from build123d import *

# Parameters (mm, degrees)
SKETCH1_W           = 66.85
SKETCH1_H           = 96.52
BOSS_EXTRUDE2_DEPTH = 3
SKETCH2_W           = 31.925
SKETCH2_H           = 3
CUT_EXTRUDE1_DEPTH  = 3
SKETCH3_W           = 48.26
SKETCH3_H           = 3
CUT_EXTRUDE2_DEPTH  = 3
SKETCH4_W           = 10.643333334
SKETCH4_H           = 3
BOSS_EXTRUDE3_DEPTH = 3
SKETCH5_W           = 16.086666666
SKETCH5_H           = 3
BOSS_EXTRUDE4_DEPTH = 3
SKETCH6_R           = 1.45
CUT_EXTRUDE10_DEPTH = 3
SKETCH7_R           = 1.45
CUT_EXTRUDE11_DEPTH = 3
SKETCH9_W           = 96.52
SKETCH9_H           = 3
BOSS_EXTRUDE5_DEPTH = 17.25
SKETCH10_W          = 12.7
SKETCH10_H          = 6.86
CUT_EXTRUDE12_DEPTH = 3
SKETCH12_W          = 15
SKETCH12_H          = 3
CUT_EXTRUDE14_DEPTH = 3


with BuildPart() as part:
    # Sketch1 → Boss-Extrude2 (new body)
    with BuildSketch(Plane(origin=(0, 0, 0), x_dir=(1, 0, 0), z_dir=(0, 1, 0))):
        Rectangle(SKETCH1_W, SKETCH1_H)
    extrude(amount=BOSS_EXTRUDE2_DEPTH)

    # Sketch2 → Cut-Extrude1 (cut)
    with BuildSketch(Plane.XY.offset(48.26)):
        with Locations((0, 1.5)):
            Rectangle(SKETCH2_W, SKETCH2_H)
    cut_extrude1 = extrude(amount=-CUT_EXTRUDE1_DEPTH, mode=Mode.SUBTRACT)

    # Mirror1: Cut-Extrude1 across plane
    add(cut_extrude1.mirror(Plane.XY), mode=Mode.SUBTRACT)

    # Sketch3 → Cut-Extrude2 (cut)
    with BuildSketch(Plane.ZY.offset(33.425)):
        with Locations((0, 1.5)):
            Rectangle(SKETCH3_W, SKETCH3_H)
    extrude(amount=-CUT_EXTRUDE2_DEPTH, mode=Mode.SUBTRACT)

    # Sketch4 → Boss-Extrude3 (add)
    with BuildSketch(Plane.XY.offset(45.26)):
        with Locations((0, 1.5)):
            Rectangle(SKETCH4_W, SKETCH4_H)
    boss_extrude3 = extrude(amount=BOSS_EXTRUDE3_DEPTH)

    # Mirror2: Boss-Extrude3 across plane
    add(boss_extrude3.mirror(Plane.XY))

    # Sketch5 → Boss-Extrude4 (add)
    with BuildSketch(Plane.ZY.offset(30.425)):
        with Locations((0, 1.5)):
            Rectangle(SKETCH5_W, SKETCH5_H)
    extrude(amount=BOSS_EXTRUDE4_DEPTH)

    # Sketch6 → Cut-Extrude10 (cut)
    with BuildSketch(Plane(origin=(0, 3, 0), x_dir=(1, 0, 0), z_dir=(0, 1, 0))):
        with Locations((-32.075, 0)):
            Circle(SKETCH6_R)
    extrude(amount=-CUT_EXTRUDE10_DEPTH, mode=Mode.SUBTRACT)

    # Sketch7 → Cut-Extrude11 (cut)
    with BuildSketch(Plane(origin=(0, 3, 0), x_dir=(1, 0, 0), z_dir=(0, 1, 0))):
        with Locations((-0.211991592, -46.91)):
            Circle(SKETCH7_R)
    cut_extrude11 = extrude(amount=-CUT_EXTRUDE11_DEPTH, mode=Mode.SUBTRACT)

    # Mirror3: Cut-Extrude11 across plane
    add(cut_extrude11.mirror(Plane.XY), mode=Mode.SUBTRACT)

    # Sketch9 → Boss-Extrude5 (add)
    with BuildSketch(Plane(origin=(33.425, 0, 0), x_dir=(0, 0, -1), z_dir=(1, 0, 0))):
        with Locations((0, 1.5)):
            Rectangle(SKETCH9_W, SKETCH9_H)
    extrude(amount=BOSS_EXTRUDE5_DEPTH)

    # Sketch10 → Cut-Extrude12 (cut)
    with BuildSketch(Plane.XZ):
        with Locations((34.325, 0)):
            Rectangle(SKETCH10_W, SKETCH10_H)
    extrude(amount=-CUT_EXTRUDE12_DEPTH, mode=Mode.SUBTRACT)

    # Sketch12 → Cut-Extrude14 (cut)
    with BuildSketch(Plane.XZ):
        with Locations((38.175, -16.76)):
            Rectangle(SKETCH12_W, SKETCH12_H)
    extrude(amount=-CUT_EXTRUDE14_DEPTH, mode=Mode.SUBTRACT)


solid = part.part
Design review of the part built by this model. Coordinates are the model's own, in mm. A direction names the side the tool comes from. Round coordinates to 2 decimals unless told otherwise and drop trailing zeros. Loops run counter-clockwise (first coordinate to the right, second up) from the corner with the lowest first, then second, coordinate; pieces in that order, holes last. Notation, with made-up numbers: (87, -29.5) -> (135, -29.5) arc R33 ccw to (135, 3.5) -> close; hole circle Ø1 at (58.25, 34.25). An arc over 180 degrees is marked (long way). Use one line per item in the form item = value. Start each with the question number.
Q1. Machinability: for faces 1 (the face through (-32, 1, 8.043)), 2 (the face through (-33.425, 2, -4)), 3 (the face through (15.962, 1, 47)), 4 (the face through (-11, 2, -45.26)), 5 (the face through (30.675, 1, -17)), which of the approach directions +Z, -Z, +X, -X, +Y, -Y give a long, thin tool a straight path to every point of the face, cutting with its end or side? Answer none if there is none.
Q2. For pin 1 Ø1.5 at (y, z) = (2, -13) entering from -X (3 decimals); pin 2 Ø2 at (x, z) = (36.5, 1) entering from +Y; pin 3 Ø1.5 at (x, y) = (10.5, 1) entering from -Z, all flat-tipped, find the tip position at first contact; note any pin that passes through.
Q3. We need section B-B on y = 1.65. State how many separate pieces and enclosed holes the cut face has, then the cut area to 3 significant figures.
Q4. Wall thickness on line 1 along X through (y, z) = (1.8, -46.91) (1 decimal); line 2 along X through (y, z) = (1.6, 0) (3 decimals); line 3 along Z through (x, y) = (33, 1): over which ranges is each line inside the solid? List them lowest first. Write a range as [from, to].
Q5. Draft analysis for pull direction X (two halves, no side actions). For faces 6 (the face through (-25, 1, 48.26)), 7 (the face through (-15.962, 1, -47)), 8 (the face through (-33.425, 1, -36)), state which applies: +X half, -X half, draft (parallel to the pull), parting line (faces both ways), or undercut.
Q6. We need section A-A on z = -46.91. Give the boundary of the cut face in (x, y) (1 decimal), then the cut area to 3 significant figures.
Calculated:
q1.face_1 = -X, +Y, -Y
q1.face_2 = +Z, -Z, -X, +Y, -Y
q1.face_3 = +Z, +Y, -Y
q1.face_4 = -Z, +Y, -Y
q1.face_5 = +Y, -Y
q2.pin_1 = -30.425
q2.pin_2 = through
q2.pin_3 = -45.26
q3.separate_pieces = 1
q3.enclosed_holes = 2
q3.area = 7,740 mm²
q4.line_1 = [-33.4, -16], [-5.3, -1.7], [1.2, 5.3], [16, 50.7]
q4.line_2 = [-30.625, 27.975], [40.675, 50.675]
q4.line_3 = [-48.26, -18.26], [-15.26, -3.43], [3.43, 48.26]
q5.face_6 = draft
q5.face_7 = undercut
q5.face_8 = -X half
q6.outline = (-33.4, 0) -> (-16, 0) -> (-16, 3) -> (-33.4, 3) -> close; (-5.3, 0) -> (-1.7, 0) -> (-1.7, 3) -> (-5.3, 3) -> close; (1.2, 0) -> (5.3, 0) -> (5.3, 3) -> (1.2, 3) -> close; (16, 0) -> (50.7, 0) -> (50.7, 3) -> (16, 3) -> close
q6.area = 180 mm²
